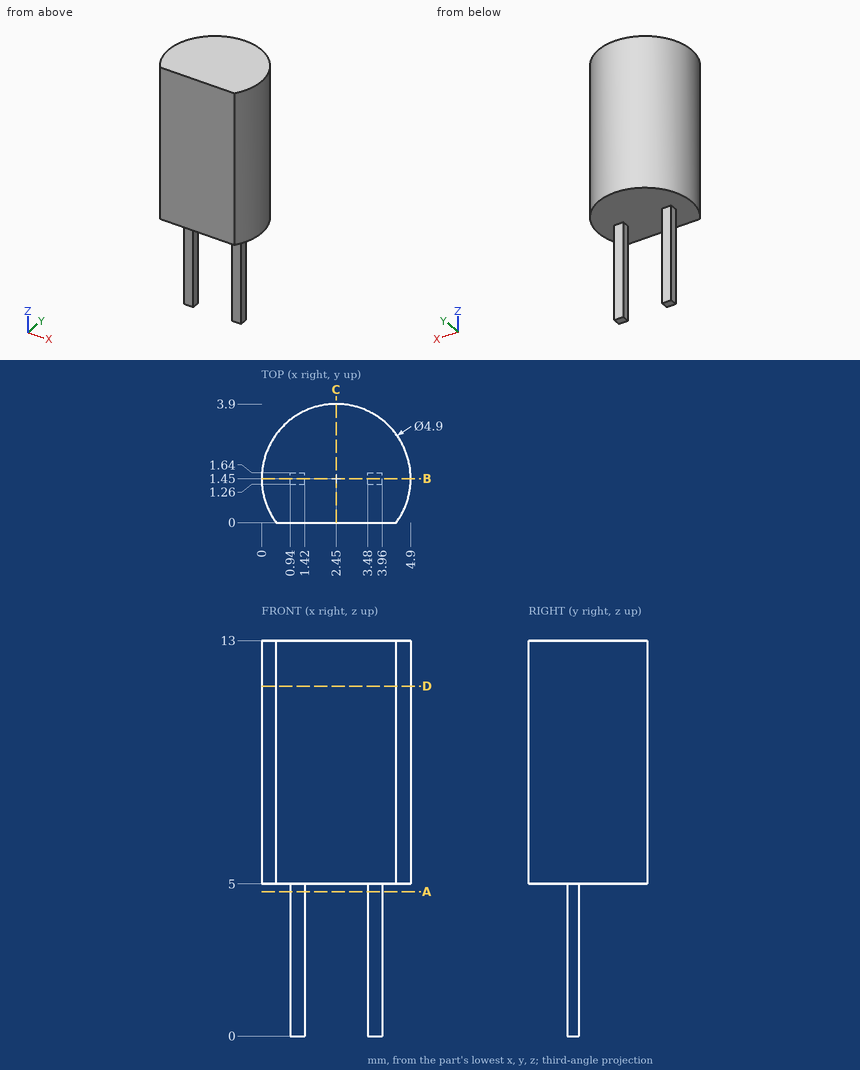
Can you work these out from the drawing? Everything is in mm from the part's minimum corner. Round coordinates to 2 decimals unless told otherwise and drop trailing zeros. Loops run counter-clockwise (first coordinate to the right, second up) from the corner with the lowest first, then second, coordinate; pieces in that order, holes last. Notation, with made-up numbers: M 53.25,86 L 65.25,86 A28 cw 65.25,115 Z; hole C -4,76 d7. An arc over 180 degrees is marked long. Answer in a Markdown table with one row per item.
1. If we section it at B-B, the plane y = 1.45: Please give me the cut outline in (x, z).
Established:
| item | result |
|---|---|
| outline | M 0,5 L 0.94,5 L 0.94,0 L 1.42,0 L 1.42,5 L 3.48,5 L 3.48,0 L 3.96,0 L 3.96,5 L 4.9,5 L 4.9,13 L 0,13 Z |
2. If we section it at C-C, the plane x = 2.45: Please give me the cut outline in (y, z), plus the area to 3 significant figures.
Established:
| item | result |
|---|---|
| outline | M 0,5 L 3.9,5 L 3.9,13 L 0,13 Z |
| area | 31.2 mm² |
3. Please list where these lines run through material, in increasing order: line 1 (Z direction, x = 0.6, y = 1.35); line 2 (X direction, y = 1.35, z = 11); line 3 (X direction, y = 3.45, z = 6). Write a range as from..to.
Established:
| item | result |
|---|---|
| line 1 | 5..13 |
| line 2 | 0..4.9 |
| line 3 | 1.03..3.87 |
4. If we section it at D-D, the plane z = 11.5: Please give me the cut outline in (x, y), plus the area to 3 significant figures.
Established:
| item | result |
|---|---|
| outline | M 0.48,0 L 4.42,0 A2.45 ccw long Z |
| area | 16.1 mm² |
5. If we section it at A-A, the plane z = 4.75: Please give me the cut outline in (x, y), plus the area to 3 significant figures.
Established:
| item | result |
|---|---|
| outline | M 0.94,1.26 L 1.42,1.26 L 1.42,1.64 L 0.94,1.64 Z; M 3.48,1.26 L 3.96,1.26 L 3.96,1.64 L 3.48,1.64 Z |
| area | 0.365 mm² |
